from build123d import *

# Parameters (mm, degrees)
F0_R     = 2.5
F0_R_2   = 4
F1_DEPTH = 5


# Not quite as in the source:
# - ends of sketch curves that miss each other by under 0.0002 mm in the source are joined


with BuildPart() as f1:
    # F0 (on Front) → F1 (new body)
    with BuildSketch(Plane.XZ):
        with BuildLine():
            ThreePointArc((215.3364533002, 370.0381469093), (202.5092928068, 283.2524328558), (215.3364530138, 196.4667187599))
            ThreePointArc((215.3364530138, 196.4667187599), (222.5589410473, 186.1945021744), (234.481309, 182.252433))
            Line((234.481309, 182.252433), (501.537276, 182.252433))
            ThreePointArc((501.537276, 182.252433), (513.4596440465, 186.1945022441), (520.6821320538, 196.4667189837))
            ThreePointArc((520.6821320538, 196.4667189837), (530.2851775529, 239.3881650909), (533.5092924377, 283.2524341717))
            ThreePointArc((533.5092924377, 283.2524341717), (530.2851774064, 327.11670224), (520.6821320538, 370.0381473561))
            ThreePointArc((520.6821320538, 370.0381473561), (513.4596440465, 380.3103637559), (501.537276, 384.252433))
            Line((501.537276, 384.252433), (234.481309, 384.252433))
            ThreePointArc((234.481309, 384.252433), (222.5589409535, 380.3103637559), (215.3364533002, 370.0381469093))
        make_face()
        with Locations((272.009293, 212.252433)):
            Circle(F0_R, mode=Mode.SUBTRACT)
        with BuildLine():
            ThreePointArc((466.4531644107, 228.2524329162), (457.7696552677, 213.8875162419), (441.958267, 208.252433))
            Line((441.958267, 208.252433), (294.060318, 208.252433))
            ThreePointArc((294.060318, 208.252433), (278.2489297323, 213.8875162419), (269.5654205893, 228.2524329162))
            ThreePointArc((269.5654205893, 228.2524329162), (264.009293, 283.252433), (269.5654212821, 338.2524329424))
            ThreePointArc((269.5654212821, 338.2524329424), (278.2489297323, 352.6173497581), (294.060318, 358.252433))
            Line((294.060318, 358.252433), (441.958267, 358.252433))
            ThreePointArc((441.958267, 358.252433), (457.7696552677, 352.6173497581), (466.4531644107, 338.2524330838))
            ThreePointArc((466.4531644107, 338.2524330838), (472.009293, 283.252433), (466.4531644107, 228.2524329162))
        make_face(mode=Mode.SUBTRACT)
        with Locations((272.009293, 354.252433)):
            Circle(F0_R, mode=Mode.SUBTRACT)
        with Locations((368.009293, 363.252433)):
            Circle(F0_R_2, mode=Mode.SUBTRACT)
        with Locations((464.009293, 212.252433)):
            Circle(F0_R, mode=Mode.SUBTRACT)
        with Locations((477.009293, 283.252433)):
            Circle(F0_R_2, mode=Mode.SUBTRACT)
        with Locations((464.009293, 354.252433)):
            Circle(F0_R, mode=Mode.SUBTRACT)
    extrude(amount=F1_DEPTH)


solid = f1.part
Input: part model. Units: mm. Frame: model coordinates. A direction names the side the tool comes from. Give positions to 0.01 mm unless a question says otherwise; leave off trailing zeros. Write each loop counter-clockwise with the first axis right and the second up, starting at its lowest first coordinate (ties: lowest second). Pieces come first, ordered by that corner, then holes. Notation, with made-up numbers: (7, -25.5) -> (41, -25.5) arc R20 cw to (41, -14.5) -> close; hole circle Ø8 at (27, 57). An arc over 180 degrees is marked (long way). Use one line per item in the form item = value. Start each with the question number.
1) Section query B-B on z = 238. Return the cut outline in (x, y), then the cut area to 3 significant figures.
2) Section query C-C on y = -2.9. Return the cut outline in (x, z).
3) Section query D-D on z = 204. Return the cut outline in (x, y).
4) Section query A-A on x = 330. Return the cut outline in (y, z), then the cut area to 3 significant figures.
5) Pin query (flat end, axial travel): pin 1 (13 mm diameter, centred on x = 368.01, z = 363.25, fed in from +Y); pin 2 (4.5 mm diameter, centred on x = 272.01, z = 354.25, fed in from +Y). Return the tip coordinate at first contact, or that it passes through.
6) Ray query, probe 1 along Z at (x, y) = (380.5, -2.25); probe 2 along X at (y, z) = (-1.7, 355); probe 3 along X at (y, z) = (-0.6, 343). Return the intervals inside material, ascending. Write a range as from..to.
7) Draft query along X for faces 1 (the cylindrical face through (478.855, -2.465, 279.704)), 2 (the cylindrical face through (222.42, -2.46, 186.3)), 3 (the cylindrical face through (513.603, -2.465, 380.203)). Return one class per face: pulls with the +X half, pulls with the -X half, needs draft (parallel to the pull), parting line crosses it, or undercut.
8) Set-up query: faces 4 (the cylindrical face through (457.955, -2.465, 214.04)), 5 (the cylindrical face through (513.32, -2.46, 186.09)). Return all of +Z, -Z, +X, -X, +Y, -Y with unobstructed straight access to the full face (end or side cutting, diameter ignored); none if empty.
Outcome:
q1.outline = (205.94, -5) -> (267.76, -5) -> (267.76, 0) -> (205.94, 0) -> close; (468.26, -5) -> (530.08, -5) -> (530.08, 0) -> (468.26, 0) -> close
q1.area = 618 mm^2
q2.outline = (215.34, 196.47) arc R20 ccw to (234.48, 182.25) -> (501.54, 182.25) arc R20 ccw to (520.68, 196.47) arc R300 ccw to (520.68, 370.04) arc R20 ccw to (501.54, 384.25) -> (234.48, 384.25) arc R20 ccw to (215.34, 370.04) arc R300 ccw to start; hole circle Ø5 at (272.01, 212.25); hole circle Ø5 at (272.01, 354.25); hole (269.57, 228.25) arc R25 ccw to (294.06, 208.25) -> (441.96, 208.25) arc R25 ccw to (466.45, 228.25) arc R275 ccw to (466.45, 338.25) arc R25 ccw to (441.96, 358.25) -> (294.06, 358.25) arc R25 ccw to (269.57, 338.25) arc R275 ccw to start; hole circle Ø8 at (368.01, 363.25); hole circle Ø5 at (464.01, 212.25); hole circle Ø5 at (464.01, 354.25); hole circle Ø8 at (477.01, 283.25)
q3.outline = (213.17, -5) -> (522.85, -5) -> (522.85, 0) -> (213.17, 0) -> close
q4.outline = (-5, 182.25) -> (0, 182.25) -> (0, 208.25) -> (-5, 208.25) -> close; (-5, 358.25) -> (0, 358.25) -> (0, 384.25) -> (-5, 384.25) -> close
q4.area = 260 mm^2
q5.pin_1 = 0
q5.pin_2 = through
q6.probe_1 = 182.25..208.25, 358.25..384.25
q6.probe_2 = 211.22..269.62, 274.39..281.73, 454.29..461.62, 466.39..524.8
q6.probe_3 = 208.52..271.04, 464.98..527.5
q7.face_1 = undercut
q7.face_2 = pulls with the -X half
q7.face_3 = pulls with the +X half
q8.face_4 = +Y, -Y
q8.face_5 = -Z, +X, +Y, -Y
